```python
from build123d import *

# Parameters (mm, degrees)
F0_W          = 100
F0_H          = 100
F1_DEPTH      = 50
F2_R          = 27
F3_DEPTH      = 100.001
F4_R          = 45
F5_DEPTH      = 23
F6_R          = 45
F6_R_2        = 27
F7_DEPTH      = 23
F8_R          = 49.99999
F9_R          = 25
F10_DEPTH     = 10
F11_R         = 26
F11_R_2       = 25
F12_DEPTH     = 105
F13_T4_DEPTH  = 100
F13_S5_R      = 26
F13_T6_DEPTH  = 63
F13_T10_DEPTH = 100
F13_S11_R     = 26
F13_T12_DEPTH = 63
F15_DEPTH     = 77.0010001


# Not quite as in the source:
# - a fillet or chamfer that OpenCascade refuses, or shapes differently, is made with other operations: its cross-section is extruded or revolved along the edge and cut away or added
# - a fillet or chamfer is up to 0.001 mm smaller than in the source, because OpenCascade refuses the exact size


with BuildPart() as f1:
    # F0 (on Front) → F1 (new body, symmetric)
    with BuildSketch(Plane.XZ):
        Rectangle(F0_W, F0_H)
    extrude(amount=F1_DEPTH, both=True)

    # F2 (on face) → F3 (cut, through all)
    with BuildSketch(Plane.XY.offset(50)):
        Circle(F2_R)
    extrude(amount=-F3_DEPTH, mode=Mode.SUBTRACT)

    # F4 (on face) → F5 (cut)
    with BuildSketch(Plane.XY.offset(50)):
        Circle(F4_R)
    extrude(amount=-F5_DEPTH, mode=Mode.SUBTRACT)

    # F6 (on face) → F7 (cut)
    with BuildSketch(Plane(origin=(0, 0, -50), x_dir=(1, 0, 0), z_dir=(0, 0, -1))):
        Circle(F6_R)
        Circle(F6_R_2, mode=Mode.SUBTRACT)
    extrude(amount=-F7_DEPTH, mode=Mode.SUBTRACT)

    # F8 (radius 50 in the source; OpenCascade refuses exactly that, so slightly less here)
    f8_edges = [f1.edges().sort_by_distance(p)[0] for p in [
        (50, -50, 0),
        (-50, -50, 0),
    ]]
    fillet(f8_edges, radius=F8_R)

    # F9 (on face) → F10 (cut)
    with BuildSketch(Plane(origin=(0, 50, 0), x_dir=(-1, 0, 0), z_dir=(0, 1, 0))):
        Circle(F9_R)
    extrude(amount=-F10_DEPTH, mode=Mode.SUBTRACT)

    # F11 (on face) → F12 (join)
    with BuildSketch(Plane(origin=(0, 50, 0), x_dir=(-1, 0, 0), z_dir=(0, 1, 0))):
        Circle(F11_R)
        Circle(F11_R_2, mode=Mode.SUBTRACT)
    extrude(amount=F12_DEPTH)

    # F13: fillet of radius 50 on 2 edges, made by hand


with BuildPart() as f13_tool2:
    # F13_s3 → F13_t4 (new body)
    with BuildSketch(Plane.XY.offset(-50)):
        with BuildLine():
            ThreePointArc((50, 0), (35.3553390593, 35.3553390593), (0, 50))
            Line((0, 50), (0, 51))
            Line((0, 51), (51, 51))
            Line((51, 51), (51, 0))
            Line((51, 0), (50, 0))
        make_face()
    extrude(amount=F13_T4_DEPTH)

    # F13_s5 → F13_t6 (cut, symmetric)
    with BuildSketch(Plane.XZ.offset(-25.5)):
        Circle(F13_S5_R)
    extrude(amount=F13_T6_DEPTH, both=True, mode=Mode.SUBTRACT)


with BuildPart() as f1_1:
    add(f1.part)

    # F13_t1: cut F13_tool2
    add(f13_tool2.part, mode=Mode.SUBTRACT)


with BuildPart() as f13_tool8:
    # F13_s9 → F13_t10 (new body)
    with BuildSketch(Plane.XY.offset(50)):
        with BuildLine():
            ThreePointArc((0, 50), (-35.3553390593, 35.3553390593), (-50, 0))
            Line((-50, 0), (-51, 0))
            Line((-51, 0), (-51, 51))
            Line((-51, 51), (0, 51))
            Line((0, 51), (0, 50))
        make_face()
    extrude(amount=-F13_T10_DEPTH)

    # F13_s11 → F13_t12 (cut, symmetric)
    with BuildSketch(Plane.XZ.offset(-25.5)):
        Circle(F13_S11_R)
    extrude(amount=F13_T12_DEPTH, both=True, mode=Mode.SUBTRACT)


with BuildPart() as f1_2:
    add(f1_1.part)

    # F13_t7: cut F13_tool8
    add(f13_tool8.part, mode=Mode.SUBTRACT)

    # F14 (on face) → F15 (cut, through all)
    with BuildSketch(Plane.XY.offset(27)):
        with BuildLine():
            ThreePointArc((-32.0062519729, 5.6435657742), (-22.9809703886, 22.9809703886), (-5.6435657742, 32.0062519729))
            Line((-5.6435657742, 32.0062519729), (-6.9459271067, 39.3923101205))
            ThreePointArc((-6.9459271067, 39.3923101205), (-28.2842712475, 28.2842712475), (-39.3923101205, 6.9459271067))
            Line((-39.3923101205, 6.9459271067), (-32.0062519729, 5.6435657742))
        make_face()
        with BuildLine():
            ThreePointArc((5.6435657742, 32.0062519729), (22.9809703886, 22.9809703886), (32.0062519729, 5.6435657742))
            Line((32.0062519729, 5.6435657742), (39.3923101205, 6.9459271067))
            ThreePointArc((39.3923101205, 6.9459271067), (28.2842712475, 28.2842712475), (6.9459271067, 39.3923101205))
            Line((6.9459271067, 39.3923101205), (5.6435657742, 32.0062519729))
        make_face()
        with BuildLine():
            Line((39.3923101205, -6.9459271067), (32.0062519729, -5.6435657742))
            ThreePointArc((32.0062519729, -5.6435657742), (22.9809703886, -22.9809703886), (5.6435657742, -32.0062519729))
            Line((5.6435657742, -32.0062519729), (6.9459271067, -39.3923101205))
            ThreePointArc((6.9459271067, -39.3923101205), (28.2842712475, -28.2842712475), (39.3923101205, -6.9459271067))
        make_face()
        with BuildLine():
            Line((-6.9459271067, -39.3923101205), (-5.6435657742, -32.0062519729))
            ThreePointArc((-5.6435657742, -32.0062519729), (-22.9809703886, -22.9809703886), (-32.0062519729, -5.6435657742))
            Line((-32.0062519729, -5.6435657742), (-39.3923101205, -6.9459271067))
            ThreePointArc((-39.3923101205, -6.9459271067), (-28.2842712475, -28.2842712475), (-6.9459271067, -39.3923101205))
        make_face()
    extrude(amount=-F15_DEPTH, mode=Mode.SUBTRACT)


solid = f1_2.part
```
Model file for the job. Use its own axes, mm. A direction names the side the tool comes from. Give positions to 0.01 mm unless a question says otherwise; leave off trailing zeros. Write each loop counter-clockwise with the first axis right and the second up, starting at its lowest first coordinate (ties: lowest second). Pieces come first, ordered by that corner, then holes. Notation, with made-up numbers: M -34.5,18.25 L 14.5,18.25 A30 cw 14.5,50.25 Z; hole C 7,10.5 d6. An arc over 180 degrees is marked long. Use a Markdown table: item, result.
1) Pin check, flat tips, straight feed: pin 1 (12 mm diameter, centred on x = -10.5, z = -23.5, fed in from -Y); pin 2 (10 mm diameter, centred on y = 122, z = 18.5, fed in from +X); pin 3 (25 mm diameter, centred on x = -8, z = 9.5, fed in from +Y). Stop position of each tip, or through.
Responses:
| item | result |
|---|---|
| pin 1 | stops at y = -49.8 |
| pin 2 | stops at x = 22.22 |
| pin 3 | stops at y = 40 |
2) Pull direction Y, two halves, no side cores. Call faces 5 (the flat face through (0, 40, 0)), 6 (the cylindrical face through (-23.846, 96.695, 7.509)), 7 (the cylindrical face through (-22.78, -23.18, 0.38)), 8 (the cylindrical face through (-35.742, -34.964, 0.7)): +Y half, -Y half, draft (parallel to the pull), parting line (faces both ways), or undercut.
Responses:
| item | result |
|---|---|
| face 5 | +Y half |
| face 6 | draft |
| face 7 | undercut |
| face 8 | -Y half |
3) Cut at D-D (y = 90.5). List the corners of the cut face in (x, z).
Responses:
| item | result |
|---|---|
| outline | C 0,0 d52; hole C 0,0 d50 |
4) Cut at C-C (z = 14.5). Give the number of separate pieces and of enclosed holes in the cut face, and give its area (3 significant figures).
Responses:
| item | result |
|---|---|
| separate pieces | 1 |
| enclosed holes | 5 |
| area | 4,150 mm2 |
5) Drill centre lines: line 1 (X direction, y = 0, z = -39); line 2 (X direction, y = 18, z = -5.5); line 3 (Z direction, x = 0, y = 122.5). Where is each one in solid material? Low to high. Write a range as from..to.
Responses:
| item | result |
|---|---|
| line 1 | x = -50..-45, 45..50 |
| line 2 | x = -46.65..-35.72, -27.06..-20.12, 20.12..27.06, 35.72..46.65 |
| line 3 | z = -26..-25, 25..26 |
6) Tool access for faces 1 (the flat face through (-6.286, 35.648, 0.378)), 2 (the flat face through (19.4, 19.4, -27)), 3 (the cylindrical face through (34.964, -35.742, 0.7)), 4 (the cylindrical face through (20.765, -39.923, 38.661)): list every direction of +Z, -Z, +X, -X, +Y, -Y with a clear straight run to the whole face (end or side of a thin tool).
Responses:
| item | result |
|---|---|
| face 1 | +Z, -Z |
| face 2 | -Z |
| face 3 | +Z, -Z, +X, -Y |
| face 4 | +Z |
7) Cut at B-B (x = -2). List the corners of the cut face in (y, z), and give its area (3 significant figures).
Responses:
| item | result |
|---|---|
| outline | M -49.96,-50 L -44.96,-50 L -44.96,-27 L -26.93,-27 L -26.93,27 L -44.96,27 L -44.96,50 L -49.96,50 Z; M 26.93,-27 L 44.96,-27 L 44.96,-50 L 49.96,-50 L 49.96,-25.92 L 155,-25.92 L 155,-24.92 L 40,-24.92 L 40,24.92 L 155,24.92 L 155,25.92 L 49.96,25.92 L 49.96,50 L 44.96,50 L 44.96,27 L 26.93,27 Z |
| area | 2,660 mm2 |
